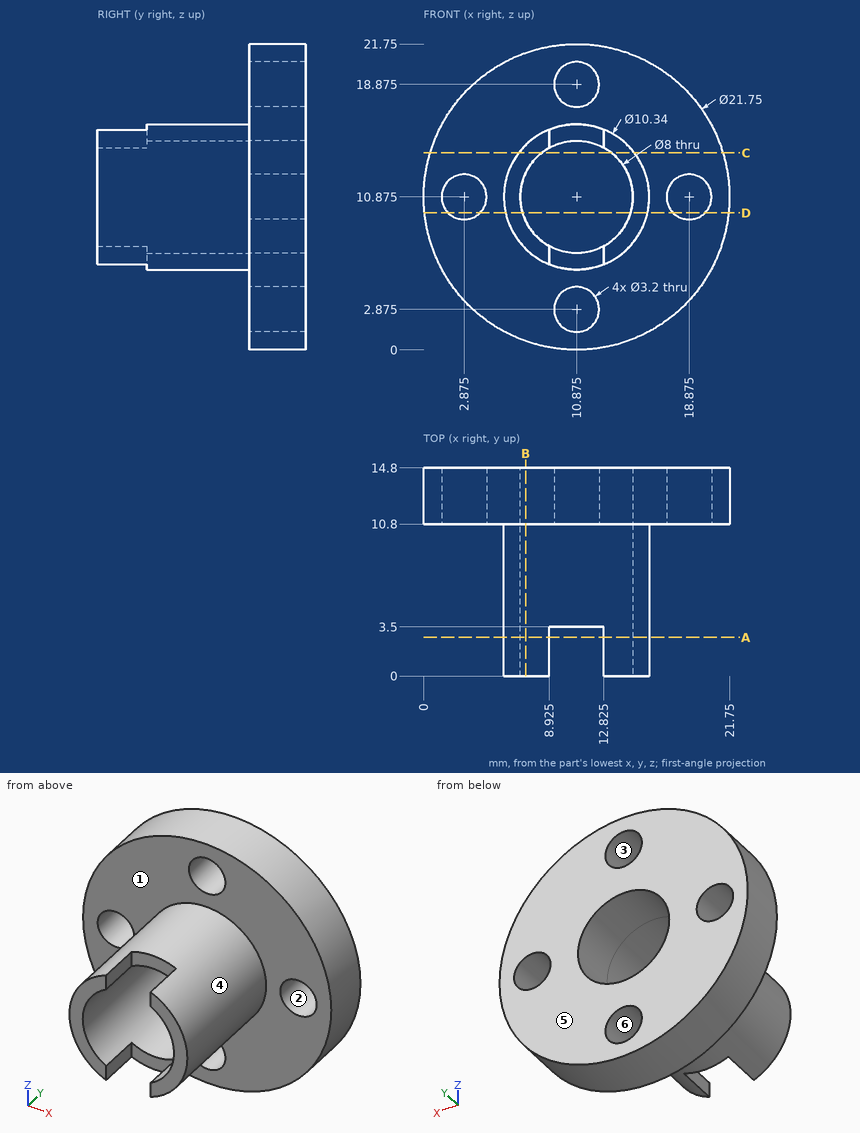
Can you work these out from the drawing? Everything is in mm from the part's minimum corner. A direction names the side the tool comes from. Coordinates: 2 decimals unless noted, no trailing zeros. Loops run counter-clockwise (first coordinate to the right, second up) from the corner with the lowest first, then second, coordinate; pieces in that order, holes last. Notation, with made-up numbers: (53.5, -31) -> (59.5, -31) arc R24 cw to (59.5, 2) -> close; hole circle Ø10 at (74, 26). An arc over 180 degrees is marked (long way). Return JSON: item names as keys, results as strings.
1) If we section it at C-C, the plane z = 14: Write out the boundary of the cut face in (x, y).
Results below:
{"outline": "(0.46, 10.8) -> (6.76, 10.8) -> (6.76, 0) -> (8.38, 0) -> (8.38, 14.8) -> (0.46, 14.8) -> close; (13.37, 0) -> (14.99, 0) -> (14.99, 10.8) -> (21.29, 10.8) -> (21.29, 14.8) -> (13.37, 14.8) -> close"}
2) Will these pins go through, and if not, where does the flat tip stop? pin 1 (0.6 mm diameter, centred on y = 2, z = 15, fed in from -X); pin 2 (1 mm diameter, centred on y = 8, z = 12.5, fed in from -X); pin 3 (1 mm diameter, centred on y = 1.5, z = 7, fed in from -X).
Results below:
{"pin 1": "x = 7.4", "pin 2": "x = 5.83", "pin 3": "x = 6.96"}
3) If we section it at A-A, the plane y = 2.75: Write out the boundary of the cut face in (x, z) (1 decimal).
Results below:
{"outline": "(8.9, 6.1) -> (8.9, 7.4) arc R4 cw to (8.9, 14.4) -> (8.9, 15.7) arc R5.2 ccw to start; (12.8, 6.1) arc R5.2 ccw to (12.8, 15.7) -> (12.8, 14.4) arc R4 cw to (12.8, 7.4) -> close"}
4) Thinking about a two-plate mould opening in Z: for the marked faces 3, 4, 5 and 6, which applies, +Z half, -Z half, draft (parallel to the pull), parting line (faces both ways), or undercut?
Results below:
{"face 3": "undercut", "face 4": "parting line", "face 5": "draft", "face 6": "undercut"}
5) If we section it at B-B, the plane x = 7.25: Write out the boundary of the cut face in (y, z).
Results below:
{"outline": "(0, 7.19) -> (10.8, 7.19) -> (10.8, 0.62) -> (14.8, 0.62) -> (14.8, 9.18) -> (0, 9.18) -> close; (0, 12.57) -> (14.8, 12.57) -> (14.8, 21.13) -> (10.8, 21.13) -> (10.8, 14.56) -> (0, 14.56) -> close"}
6) For the marked faces 1 and 2, which set-ups out of +Z, -Z, +X, -X, +Y, -Y let a thin tool reach every point of the face, with its end or its side?
Results below:
{"face 1": "-Y", "face 2": "+Y, -Y"}
7) I need wall thicknesses on line 1 (Y direction, x = 7.5, z = 17); line 2 (X direction, y = 12.5, z = 2.5); line 3 (X direction, y = 12.25, z = 2.75). Which ranges of each line are inside material? Lowest first, please. Write a range as from..to.
Results below:
{"line 1": "10.8..14.8", "line 2": "3.94..9.32, 12.43..17.81", "line 3": "3.65..9.28, 12.47..18.1"}
8) If we section it at D-D, the plane z = 9.75: Write out the boundary of the cut face in (x, y).
Results below:
{"outline": "(0.06, 10.8) -> (1.74, 10.8) -> (1.74, 14.8) -> (0.06, 14.8) -> close; (4.01, 10.8) -> (5.83, 10.8) -> (5.83, 0) -> (7.04, 0) -> (7.04, 14.8) -> (4.01, 14.8) -> close; (14.71, 0) -> (15.92, 0) -> (15.92, 10.8) -> (17.74, 10.8) -> (17.74, 14.8) -> (14.71, 14.8) -> close; (20.01, 10.8) -> (21.69, 10.8) -> (21.69, 14.8) -> (20.01, 14.8) -> close"}
